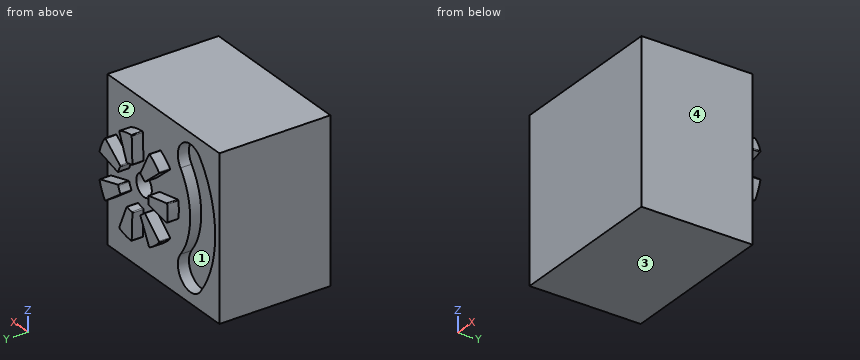
```python
from build123d import *

# Parameters (mm, degrees)
SKETCH1_W           = 92.075
SKETCH1_H           = 92.075
BOSS_EXTRUDE1_DEPTH = 63.5
CUT_EXTRUDE1_DEPTH  = 6.35
BOSS_EXTRUDE2_DEPTH = 6.35
SKETCH5_R           = 6.35
CUT_EXTRUDE2_DEPTH  = 19.05


with BuildPart() as part:
    # Sketch1 → Boss-Extrude1 (new body)
    with BuildSketch(Plane(origin=(0, 0, 0), x_dir=(1, 0, 0), z_dir=(0, 1, 0))):
        Rectangle(SKETCH1_W, SKETCH1_H)
    extrude(amount=-BOSS_EXTRUDE1_DEPTH)

    # Sketch3 → Cut-Extrude1 (cut)
    with BuildSketch(Plane(origin=(0, 0, 0), x_dir=(1, 0, 0), z_dir=(0, 1, 0))):
        with BuildLine():
            ThreePointArc((-14.063201547, 23.287775446), (-15.921775446, 37.752798453), (-30.386798453, 35.894224554))
            ThreePointArc((-30.386798453, 35.894224554), (-42.633573767, 0), (-30.386798453, -35.894224554))
            ThreePointArc((-30.386798453, -35.894224554), (-15.921775446, -37.752798453), (-14.063201547, -23.287775446))
            ThreePointArc((-14.063201547, -23.287775446), (-22.008773767, 0), (-14.063201547, 23.287775446))
        make_face()
    extrude(amount=-CUT_EXTRUDE1_DEPTH, mode=Mode.SUBTRACT)

    # Sketch4 → Boss-Extrude2 (add)
    with BuildSketch(Plane(origin=(0, 0, 0), x_dir=(1, 0, 0), z_dir=(0, 1, 0))):
        with BuildLine():
            Line((42.981199166, 7.263084177), (28.623508469, 3.415952549))
            ThreePointArc((28.623508469, 3.415952549), (28.246537351, 3.461897832), (28.006758071, 3.756387374))
            ThreePointArc((28.006758071, 3.756387374), (27.317235926, 5.510466133), (26.375711245, 7.143182998))
            ThreePointArc((26.375711245, 7.143182998), (26.294960734, 7.5142592), (26.49406885, 7.837638468))
            Line((26.49406885, 7.837638468), (38.453531121, 16.664583926))
            ThreePointArc((38.453531121, 16.664583926), (38.835445953, 16.757478046), (39.169323269, 16.550079409))
            ThreePointArc((39.169323269, 16.550079409), (41.620030834, 12.3985488), (43.337949301, 7.894114306))
            ThreePointArc((43.337949301, 7.894114306), (43.291940716, 7.503766427), (42.981199166, 7.263084177))
        make_face()
        with BuildLine():
            Line((27.096930878, 25.720938792), (21.152865774, 12.096996853))
            ThreePointArc((21.152865774, 12.096996853), (20.881906657, 11.830915381), (20.502165527, 11.827059617))
            ThreePointArc((20.502165527, 11.827059617), (18.700861504, 12.381619715), (16.837321021, 12.663488392))
            ThreePointArc((16.837321021, 12.663488392), (16.496854843, 12.831717328), (16.368168631, 13.189009997))
            Line((16.368168631, 13.189009997), (16.923587539, 28.042804588))
            ThreePointArc((16.923587539, 28.042804588), (17.089079994, 28.399316164), (17.45939988, 28.531041026))
            ThreePointArc((17.45939988, 28.531041026), (22.233188385, 27.858644358), (26.826001728, 26.39329813))
            ThreePointArc((26.826001728, 26.39329813), (27.102502105, 26.113949248), (27.096930878, 25.720938792))
        make_face()
        with BuildLine():
            Line((2.762319753, 24.810401886), (9.707882502, 11.668755794))
            ThreePointArc((9.707882502, 11.668755794), (9.746973129, 11.291012341), (9.513222964, 10.991714741))
            ThreePointArc((9.513222964, 10.991714741), (7.956555733, 9.929161112), (6.57428344, 8.647928739))
            ThreePointArc((6.57428344, 8.647928739), (6.230479572, 8.486630588), (5.870902373, 8.608787991))
            Line((5.870902373, 8.608787991), (-5.395963847, 18.304221426))
            ThreePointArc((-5.395963847, 18.304221426), (-5.571512963, 18.65588997), (-5.443608935, 19.027546823))
            ThreePointArc((-5.443608935, 19.027546823), (-1.941499602, 22.340612501), (2.067726493, 25.017790136))
            ThreePointArc((2.067726493, 25.017790136), (2.458525409, 25.059795657), (2.762319753, 24.810401886))
        make_face()
        with BuildLine():
            Line((-11.698175696, 5.21712632), (2.906864493, 2.453703622))
            ThreePointArc((2.906864493, 2.453703622), (3.226568823, 2.248746714), (3.314828266, 1.879384474))
            ThreePointArc((3.314828266, 1.879384474), (3.175000001, -0.000158326), (3.314875129, -1.87969764))
            ThreePointArc((3.314875129, -1.87969764), (3.226624896, -2.24906208), (2.906925676, -2.454026959))
            Line((2.906925676, -2.454026959), (-11.698045607, -5.217813808))
            ThreePointArc((-11.698045607, -5.217813808), (-12.08244423, -5.135801882), (-12.293270401, -4.804078229))
            ThreePointArc((-12.293270401, -4.804078229), (-12.699999998, -0.000356234), (-12.293390173, 4.803375901))
            ThreePointArc((-12.293390173, 4.803375901), (-12.082572273, 5.13510481), (-11.698175696, 5.21712632))
        make_face()
        with BuildLine():
            Line((-5.395507456, -18.304751776), (5.871117022, -8.609037424))
            ThreePointArc((5.871117022, -8.609037424), (6.230691175, -8.486871055), (6.574499064, -8.648160634))
            ThreePointArc((6.574499064, -8.648160634), (7.956803301, -9.929358541), (9.513497025, -10.991873357))
            ThreePointArc((9.513497025, -10.991873357), (9.747254652, -11.291165129), (9.708173444, -11.668909556))
            Line((9.708173444, -11.668909556), (2.762938362, -24.81072882))
            ThreePointArc((2.762938362, -24.81072882), (2.459150236, -25.060130166), (2.068350273, -25.018134389))
            ThreePointArc((2.068350273, -25.018134389), (-1.940942572, -22.341056718), (-5.443134509, -19.02807836))
            ThreePointArc((-5.443134509, -19.02807836), (-5.571047804, -18.656424696), (-5.395507456, -18.304751776))
        make_face()
        with BuildLine():
            Line((16.924286738, -28.042778435), (16.368497476, -13.188997697))
            ThreePointArc((16.368497476, -13.188997697), (16.49717478, -12.831701819), (16.837636763, -12.663464394))
            ThreePointArc((16.837636763, -12.663464394), (18.701170218, -12.381549253), (20.502460413, -11.826944243))
            ThreePointArc((20.502460413, -11.826944243), (20.882201639, -11.830790538), (21.15316739, -12.096865255))
            Line((21.15316739, -12.096865255), (27.097572182, -25.720658985))
            ThreePointArc((27.097572182, -25.720658985), (27.103153208, -26.113669301), (26.826659795, -26.393025077))
            ThreePointArc((26.826659795, -26.393025077), (22.23388299, -27.858485819), (17.460111251, -28.531001513))
            ThreePointArc((17.460111251, -28.531001513), (17.089788082, -28.399285884), (16.924286738, -28.042778435))
        make_face()
        with BuildLine():
            Line((38.453946616, -16.664020964), (26.494264265, -7.837373698))
            ThreePointArc((26.494264265, -7.837373698), (26.295148086, -7.513999394), (26.375889345, -7.142921178))
            ThreePointArc((26.375889345, -7.142921178), (27.317373317, -5.510180839), (28.006851726, -3.756084888))
            ThreePointArc((28.006851726, -3.756084888), (28.246623663, -3.461589368), (28.623593636, -3.415634686))
            Line((28.623593636, -3.415634686), (42.98138025, -7.262408328))
            ThreePointArc((42.98138025, -7.262408328), (43.292127801, -7.503082831), (43.338146119, -7.893429562))
            ThreePointArc((43.338146119, -7.893429562), (41.620339963, -12.397906888), (39.169735909, -16.549498601))
            ThreePointArc((39.169735909, -16.549498601), (38.835863765, -16.756905562), (38.453946616, -16.664020964))
        make_face()
    extrude(amount=BOSS_EXTRUDE2_DEPTH)

    # Sketch5 → Cut-Extrude2 (cut)
    with BuildSketch(Plane(origin=(0, 0, 0), x_dir=(1, 0, 0), z_dir=(0, 1, 0))):
        with Locations((15.875, 0)):
            Circle(SKETCH5_R)
    extrude(amount=-CUT_EXTRUDE2_DEPTH, mode=Mode.SUBTRACT)


solid = part.part
```
For this review, take the finished solid that the model builds, in its own axes (mm). Face numbers are marked on the shaded views. Coordinates: 2 decimals unless noted, no trailing zeros. Loops run counter-clockwise (first coordinate to the right, second up) from the corner with the lowest first, then second, coordinate; pieces in that order, holes last.
1. Add section D-D, the plane z = -21. Give the boundary of the cut face in (x, y), then the cut area to 3 significant figures.
2. Add section B-B, the plane x = -36. Give the boundary of the cut face in (y, z).
3. Add section C-C, the plane x = 36.5. Give the boundary of the cut face in (y, z).
4. Mouldability with a two-part tool opening along X and no side actions: class the marked faces 1, 2, 3 and 4 as +X half, -X half, draft (parallel to the pull), parting line (faces both ways), or undercut.
5. For line 1 (X direction, y = -12.5, z = 0) (1 decimal); line 2 (Y direction, x = -13, z = -22.5); line 3 (Z direction, x = 21, y = -7.5), list the stretches that pass through material, from the lowest coordinate up.
6. Insertion check: P1, Ø4, axis at x = 15, z = -2, coming from the +Y side. The pin has a flat end and moves straight along its axis. Give the tip position at first contact, or say it passes through.
Result:
1. outline: (-46.04, -63.5) - (46.04, -63.5) - (46.04, 0) - (25.04, 0) - (25.04, 6.35) - (16.66, 6.35) - (16.66, 0) - (4.78, 0) - (4.78, 6.35) - (-3.5, 6.35) - (-3.5, 0) - (-15.7, 0) - (-15.7, -6.35) - (-38.75, -6.35) - (-38.75, 0) - (-46.04, 0) - close
1. area: 5,810 mm2
2. outline: (-63.5, -46.04) - (0, -46.04) - (0, -27.11) - (-6.35, -27.11) - (-6.35, 27.11) - (0, 27.11) - (0, 46.04) - (-63.5, 46.04) - close
3. outline: (-63.5, -46.04) - (0, -46.04) - (0, -15.22) - (6.35, -15.22) - (6.35, -5.53) - (0, -5.53) - (0, 5.53) - (6.35, 5.53) - (6.35, 15.22) - (0, 15.22) - (0, 46.04) - (-63.5, 46.04) - close
4. face 1: undercut
4. face 2: undercut
4. face 3: draft
4. face 4: +X half
5. line 1: x = -46 to 9.5, 22.2 to 46
5. line 2: y = -63.5 to 0
5. line 3: z = -46.04 to -3.75, 3.75 to 46.04
6. P1: stops at y = -19.05
